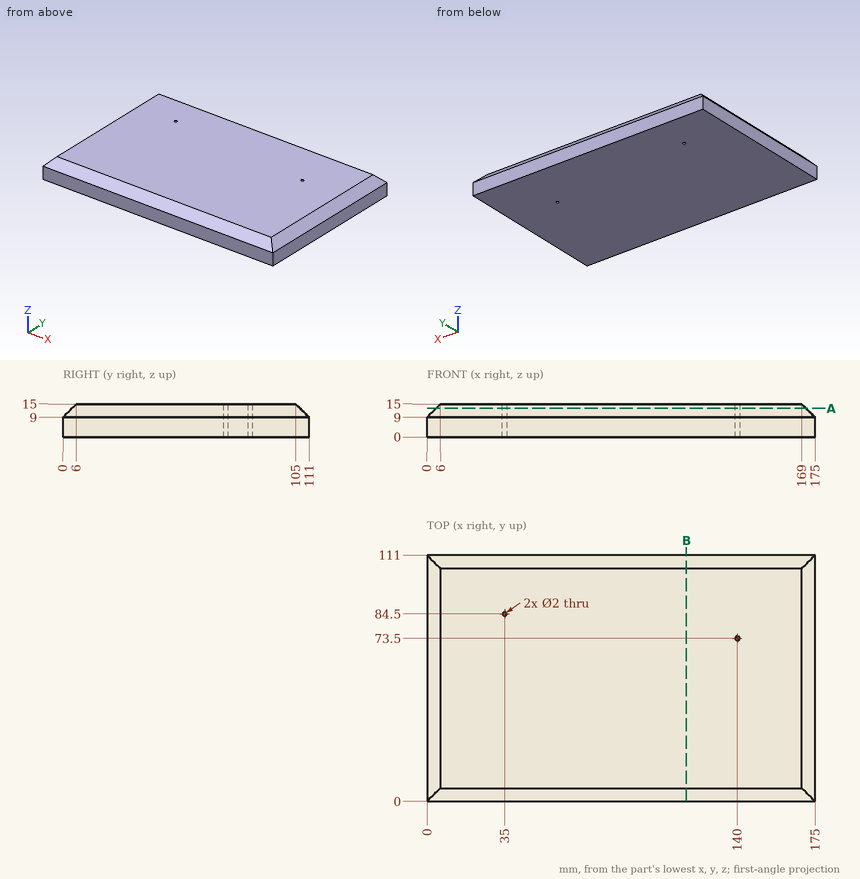
Here's the drawing with two shaded views (mm, measured from the low corner). I have some questions. Round coordinates to 2 decimals unless told otherwise and drop trailing zeros. Order: outer loops, then holes, each group sorted by start corner. A loop starts at its lowest first (then second) coordinate and runs counter-clockwise, first axis right, second up. Notation, with made-up numbers: (58.25, -14) -> (89.25, -14) arc R14 cw to (89.25, -4) -> close; hole circle Ø3 at (86, 55). An arc over 180 degrees is marked (long way). Write each question's results on one line, items separated by ' | '. Start each with the question number.
Item 1: Please list where these lines run through material, in increasing order: L1, parallel to X at y = 73.5, z = 5.75; L2, parallel to X at y = 84.5, z = 4; L3, parallel to Y at x = 35, z = 6.5.
Item 2: If we section it at A-A, the plane z = 13: Write out the boundary of the cut face in (x, y).
Item 3: Will these pins go through, and if not, where does the flat tip stop? pin 1 (8 mm diameter, centred on x = 128, z = 6.5, fed in from -Y); pin 2 (1.6 mm diameter, centred on x = 140, y = 73.5, fed in from +Z); pin 3 (4 mm diameter, centred on x = 97, z = 13.5, fed in from +Y).
Item 4: If we section it at B-B, the plane x = 117: Write out the boundary of the cut face in (y, z), then the cut area to 3 significant figures.
Results:
1) L1: x = 0 to 139, 141 to 175 | L2: x = 0 to 34, 36 to 175 | L3: y = 0 to 83.5, 85.5 to 111
2) outline: (4, 4) -> (171, 4) -> (171, 107) -> (4, 107) -> close; hole circle Ø2 at (35, 84.5); hole circle Ø2 at (140, 73.5)
3) pin 1: stops at y = 0 | pin 2: passes through | pin 3: stops at y = 108.5
4) outline: (0, 0) -> (111, 0) -> (111, 9) -> (105, 15) -> (6, 15) -> (0, 9) -> close | area: 1,630 mm2
